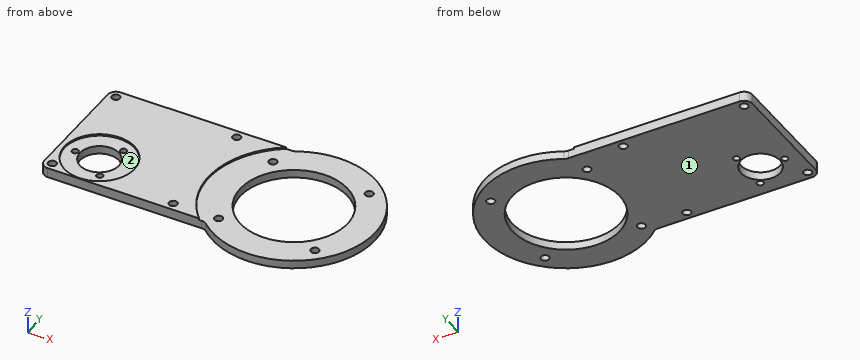
from build123d import *

# Parameters (mm, degrees)
EXTRUSION1_DEPTH                 = 12
ENL_V_START                      = -2
ENL_V_MAT_EXTRU_1_DEPTH          = 2
ESQUISSE3_R                      = 43
ENL_V_MAT_EXTRU_2_DEPTH          = 2
DIAM_TRE_DU_PER_AGE_M10_0_10_1_D = 10
DIAM_TRE_DU_PER_AGE_M10_0_10_2_D = 10
DIAM_TRE_DU_PER_AGE_M10_0_10_3_D = 10
DIAM_TRE_DU_PER_AGE_M10_0_10_4_D = 10
PER_AGE1_D                       = 132
DIAM_TRE_DU_PER_AGE_M10_0_10_5_D = 10
DIAM_TRE_DU_PER_AGE_M10_0_10_6_D = 10
DIAM_TRE_DU_PER_AGE_M8_0_8_1_D   = 8
DIAM_TRE_DU_PER_AGE_M8_0_8_2_D   = 8
DIAM_TRE_DU_PER_AGE_M8_0_8_3_D   = 8
D_GAGEMENT_M421_D                = 48
DIAM_TRE_DU_PER_AGE_M10_0_10_7_D = 10
DIAM_TRE_DU_PER_AGE_M10_0_10_8_D = 10


with BuildPart() as part:
    # Esquisse1 → Extrusion1 (new body)
    with BuildSketch(Plane(origin=(0, 0, 0), x_dir=(-1, 0, 0), z_dir=(0, 0, -1))):
        with BuildLine():
            Line((73.321211119, -72), (263, -72))
            ThreePointArc((263, -72), (270.071067812, -69.071067812), (273, -62))
            Line((273, -62), (273, 77))
            ThreePointArc((273, 77), (270.071067812, 84.071067812), (263, 87))
            Line((263, 87), (51.874849397, 87))
            ThreePointArc((51.874849397, 87), (49.443987223, 87.29995314), (47.158953998, 88.181818182))
            ThreePointArc((47.158953998, 88.181818182), (-99.289889427, -11.896127843), (66.655646472, -74.545454545))
            ThreePointArc((66.655646472, -74.545454545), (69.753680779, -72.65801267), (73.321211119, -72))
        make_face()
    extrude(amount=-EXTRUSION1_DEPTH)

    # Esquisse2 → Enlèv. mat.-Extru.1 (cut)
    with BuildSketch(Plane.XY.offset(12).offset(ENL_V_START)):
        with BuildLine():
            Line((-51.874849397, 87), (-58.787753827, 87))
            ThreePointArc((-58.787753827, 87), (-104.359806581, 11.577165901), (-76.426435217, -72))
            Line((-76.426435217, -72), (-73.321211119, -72))
            ThreePointArc((-73.321211119, -72), (-69.753680779, -72.65801267), (-66.655646472, -74.545454545))
            ThreePointArc((-66.655646472, -74.545454545), (99.289889427, -11.896127843), (-47.158953998, 88.181818182))
            ThreePointArc((-47.158953998, 88.181818182), (-49.443987223, 87.29995314), (-51.874849397, 87))
        make_face()
    extrude(amount=ENL_V_MAT_EXTRU_1_DEPTH, mode=Mode.SUBTRACT)

    # Esquisse3 → Enlèv. mat.-Extru.2 (cut)
    with BuildSketch(Plane.XY.offset(12)):
        with Locations(Location((-224, -28, 0), (0, 0, 180))):
            Circle(ESQUISSE3_R)
    extrude(amount=-ENL_V_MAT_EXTRU_2_DEPTH, mode=Mode.SUBTRACT)

    # Diamètre du perçage M10.0 (10)1 (through all)
    with Locations(Plane.XY.offset(10)):
        with Locations((59.39696962, -59.39696962)):
            Hole(DIAM_TRE_DU_PER_AGE_M10_0_10_1_D / 2)

    # Diamètre du perçage M10.0 (10)2 (through all)
    with Locations(Plane.XY.offset(10)):
        with Locations((59.39696962, 59.39696962)):
            Hole(DIAM_TRE_DU_PER_AGE_M10_0_10_2_D / 2)

    # Diamètre du perçage M10.0 (10)3 (through all)
    with Locations(Plane.XY.offset(12)):
        with Locations((-114, 77)):
            Hole(DIAM_TRE_DU_PER_AGE_M10_0_10_3_D / 2)

    # Diamètre du perçage M10.0 (10)4 (through all)
    with Locations(Plane.XY.offset(10)):
        with Locations((-59.39696962, 59.39696962)):
            Hole(DIAM_TRE_DU_PER_AGE_M10_0_10_4_D / 2)

    # Perçage1 (through all)
    with Locations(Plane.XY.offset(10)):
        with Locations((0, 0)):
            Hole(PER_AGE1_D / 2)

    # Diamètre du perçage M10.0 (10)5 (through all)
    with Locations(Plane.XY.offset(10)):
        with Locations((-59.39696962, -59.39696962)):
            Hole(DIAM_TRE_DU_PER_AGE_M10_0_10_5_D / 2)

    # Diamètre du perçage M10.0 (10)6 (through all)
    with Locations(Plane.XY.offset(12)):
        with Locations((-114, -62)):
            Hole(DIAM_TRE_DU_PER_AGE_M10_0_10_6_D / 2)

    # Diamètre du perçage M8.0 (8)1 (through all)
    with Locations(Plane.XY.offset(10)):
        with Locations((-209, -2.019237886)):
            Hole(DIAM_TRE_DU_PER_AGE_M8_0_8_1_D / 2)

    # Diamètre du perçage M8.0 (8)2 (through all)
    with Locations(Plane.XY.offset(10)):
        with Locations((-254, -28)):
            Hole(DIAM_TRE_DU_PER_AGE_M8_0_8_2_D / 2)

    # Diamètre du perçage M8.0 (8)3 (through all)
    with Locations(Plane.XY.offset(10)):
        with Locations((-209, -53.980762114)):
            Hole(DIAM_TRE_DU_PER_AGE_M8_0_8_3_D / 2)

    # Dégagement M421 (through all)
    with Locations(Plane.XY.offset(10)):
        with Locations((-224, -28)):
            Hole(D_GAGEMENT_M421_D / 2)

    # Diamètre du perçage M10.0 (10)7 (through all)
    with Locations(Plane.XY.offset(12)):
        with Locations((-263, -62)):
            Hole(DIAM_TRE_DU_PER_AGE_M10_0_10_7_D / 2)

    # Diamètre du perçage M10.0 (10)8 (through all)
    with Locations(Plane.XY.offset(12)):
        with Locations((-263, 77)):
            Hole(DIAM_TRE_DU_PER_AGE_M10_0_10_8_D / 2)


solid = part.part
Input: part model. Units: mm. Frame: model coordinates. Face numbers are marked on the shaded views. Give positions to 0.01 mm unless a question says otherwise; leave off trailing zeros. Write each loop counter-clockwise with the first axis right and the second up, starting at its lowest first coordinate (ties: lowest second). Pieces come first, ordered by that corner, then holes. Notation, with made-up numbers: M 60,43.5 L 86,43.5 A8 ccw 86,51.5 Z; hole C 3,57.25 d2. An arc over 180 degrees is marked long. Write item = value, one per line. Start each with the question number.
1) Draft query along X for the marked faces 1 and 2. Return one class per face: +X half, -X half, draft (parallel to the pull), parting line (faces both ways), or undercut.
2) First-contact query: pin 1 Ø6 at (x, y) = (-114, -62) entering from -Z; pin 2 Ø4 at (y, z) = (-65.5, 9.5) entering from -X; pin 3 Ø16 at (x, y) = (59.4, -59.4) entering from +Z; pin 4 Ø4 at (y, z) = (78.5, 3.5) entering from +X. Flat tips, straight axial feed; report the tip coordinate or a pass-through.
3) Cut plane B-B on x = -114. Return the cut outline in (y, z).
4) Material intervals for line 1 along Y through (x, z) = (-224, 4.75); line 2 along Y through (x, z) = (-114, 6.5); line 3 along Y through (x, z) = (0, 3), sorted ascending. Write a range as [from, to].
5) Cut plane D-D on z = 5.25. Count the separate pieces of the cut face and the enclosed holes in it, then the cut area to 3 significant figures.
6) Cut plane C-C on y = -28. Return the cut outline in (x, z), then the cut area to 3 significant figures.
7) Cut plane A-A on x = -224. Return the cut outline in (y, z), then the cut area to 3 significant figures.
Solved:
q1.face_1 = draft
q1.face_2 = undercut
q2.pin_1 = through
q2.pin_2 = -272.89
q2.pin_3 = 10
q2.pin_4 = 64.4
q3.outline = M -72,0 L -67,0 L -67,12 L -72,12 Z; M -57,0 L 72,0 L 72,12 L -57,12 Z; M 82,0 L 87,0 L 87,12 L 82,12 Z
q4.line_1 = [-72, -52], [-4, 87]
q4.line_2 = [-72, -67], [-57, 72], [82, 87]
q4.line_3 = [-100, -66], [66, 100]
q5.separate_pieces = 1
q5.enclosed_holes = 13
q5.area = 44,600 mm2
q6.outline = M -273,0 L -258,0 L -258,10 L -267,10 L -267,12 L -273,12 Z; M -250,0 L -248,0 L -248,10 L -250,10 Z; M -200,0 L -59.77,0 L -59.77,10 L -101.2,10 L -101.2,12 L -181,12 L -181,10 L -200,10 Z; M 59.77,0 L 96,0 L 96,10 L 59.77,10 Z
q6.area = 2,110 mm2
q7.outline = M -72,0 L -52,0 L -52,10 L -71,10 L -71,12 L -72,12 Z; M -4,0 L 87,0 L 87,12 L 15,12 L 15,10 L -4,10 Z
q7.area = 1,260 mm2
